Part model, mm, in its own coordinate system. A direction names the side the tool comes from. Give positions to 0.01 mm unless a question says otherwise; leave off trailing zeros. Order: outer loops, then holes, each group sorted by start corner. A loop starts at its lowest first (then second) coordinate and runs counter-clockwise, first axis right, second up. Notation, with made-up numbers: (7, -3) - (19, -3) arc R15 cw to (19, 8) - close; hole circle Ø2 at (71.5, 9.25). An arc over 180 degrees is marked (long way). Use a Markdown table: item, result. Add a question column.
Autodesk Inventor part; units mm, degrees
ref_plane "YZ Plane" through (0, 0, 0) normal (1, 0, 0) x (0, 1, 0)
ref_plane "XZ Plane" through (0, 0, 0) normal (0, 1, 0) x (-1, 0, 0)
ref_plane "XY Plane" through (0, 0, 0) normal (0, 0, 1) x (1, 0, 0)
sketch "Sketch1" plane through (0, 0, 0) normal (0, 0, 1) x (1, 0, 0)
  line L0 (0, 0) -> (19.4056, 0)
  line L1 (0, 0) -> (0, 19.05)
  line L2 (0, 19.05) -> (3.175, 19.05)
  line L3 (3.175, 0) -> (3.175, 3.175)
  line L4 (3.175, 3.175) -> (3.175, 19.05)
  line L5 (3.175, 3.175) -> (9.6266, 3.175)
  line L6 (9.6266, 3.175) -> (9.6266, 0)
  line L7 (19.2532, 0) -> (19.2532, 19.05)
  line L8 (19.2532, 19.05) -> (16.0782, 19.05)
  line L9 (16.0782, 3.175) -> (16.0782, 19.05)
  line L10 (16.0782, 3.175) -> (9.6266, 3.175)
  dimension "d0" = 19.4056
  dimension "d1" = 19.05
  dimension "d2" = 3.175
  dimension "d4" = 3.175
  dimension "d5" = 6.4516
extrude "Extrusion1" add sketch "Sketch1" along normal blind 12.7
sketch "Sketch2" plane through (3.175, 3.175, 0) normal (0, 1, 0) x (1, 0, 0)
  line L0 (12.9032, 0) -> (0, 0)
  line L1 (0, 0) -> (0, -12.7)
  line L2 (12.9032, -12.7) -> (0, -12.7)
  line L3 (12.9032, 0) -> (12.9032, -12.7)
  line L4 (0, 0) -> (6.4516, 0)
  line L5 (12.9032, 0) -> (0, 0)
  line L6 (6.4516, 0) -> (6.4516, -6.35)
  circle A0 centre (6.4516, -6.35) radius 2.3241
  point P0 (-3.175, 0)
  dimension "d8" = 6.4516
  dimension "d9" = 6.35
  dimension "d10" = 4.6482
extrude "Extrusion2" cut sketch "Sketch2" against normal blind 12.7 contours A0
chamfer "Chamfer1" distance 1.5875 angle 45 4 edges at (1.5875, 19.05, 0) (1.5875, 19.05, 12.7) (17.6657, 19.05, 12.7) (17.6657, 19.05, 0)
sketch "Sketch3" plane through (19.2532, 0, 12.7) normal (1, 0, 0) x (0, 0, -1)
  line L0 (11.1125, 19.05) -> (12.7, 17.4625)
  line L1 (11.1125, 19.05) -> (1.5875, 19.05)
  line L2 (0, 17.4625) -> (1.5875, 19.05)
  line L3 (0, 0) -> (0, 17.4625)
  line L4 (12.7, 0) -> (0, 0)
  line L5 (12.7, 0) -> (12.7, 17.4625)
  line L6 (12.7, 0) -> (0, 0)
  line L7 (12.7, 0) -> (6.35, 0)
  line L8 (6.35, 0) -> (6.35, 12.7)
  circle A0 centre (6.35, 12.7) radius 2.3241
  dimension "d16" = 6.35
  dimension "d17" = 12.7
  dimension "d18" = 4.6482
extrude "Extrusion3" cut sketch "Sketch3" against normal through all contours A0
fillet "Fillet1" radius 1.27 4 edges at (3.175, 3.175, 6.35) (16.0782, 3.175, 6.35) (19.2532, 0, 6.35) (0, 0, 6.35)
properties part number "U Bracket"
1. Tool access for faces 1 (the face through (19.253, 10, 6)), 2 (the face through (16.078, 10, 6)): list every direction of +Z, -Z, +X, -X, +Y, -Y with a clear straight run to the whole face (end or side of a thin tool).
2. Cut at C-C (y = 12.7). Write the cut outline in (x, z) (3 decimals), plus the area to 3 significant figures.
3. Drill centre lines: probe 1 along X at (y, z) = (9, 2.75) (3 decimals); probe 2 along Z at (x, y) = (17.3, 12.7); probe 3 along Y at (x, z) = (17.3, 6.35). Where is each one in solid material? Low to high. Write a range as [from, to].
4. Mould opens along Z. For faces 3 (the face through (17.688, 18.267, 0.805)), 4 (the face through (18, 19.05, 6)), 5 (the face through (1.61, 10.43, 6.85)), 6 (the face through (9.12, 1.61, 8.62)) say: released by +Z, released by -Z, zero draft, split by the parting line, or undercut.
5. Cut at A-A (z = 6.35). State how many separate pieces and enclosed holes the cut face has, plus the area to 3 significant figures.
6. Cut at B-B (y = 5.75). Write the cut outline in (x, z) (3 decimals).
7. Pin check, flat tip, straight feed: P1, Ø4, axis at y = 12.7, z = 6.35, coming from the -X side. Stop position of the tip, or through.
8. Cut at D-D (x = 8.5). Write the cut outline in (y, z) (3 decimals).
Responses:
| question | item | result |
|---|---|---|
| 1 | face 1 | +Z, -Z, +X, +Y, -Y |
| 1 | face 2 | +Z, -Z, +Y |
| 2 | outline | (0, 0) - (3.175, 0) - (3.175, 4.026) - (0, 4.026) - close; (0, 8.674) - (3.175, 8.674) - (3.175, 12.7) - (0, 12.7) - close; (16.078, 0) - (19.253, 0) - (19.253, 4.026) - (16.078, 4.026) - close; (16.078, 8.674) - (19.253, 8.674) - (19.253, 12.7) - (16.078, 12.7) - close |
| 2 | area | 51.1 mm² |
| 3 | probe 1 | x = [0, 3.175], [16.078, 19.253] |
| 3 | probe 2 | z = [0, 4.03], [8.67, 12.7] |
| 3 | probe 3 | y = [0, 10.38], [15.02, 19.05] |
| 4 | face 3 | released by -Z |
| 4 | face 4 | zero draft |
| 4 | face 5 | undercut |
| 4 | face 6 | undercut |
| 5 | separate pieces | 4 |
| 5 | enclosed holes | 0 |
| 5 | area | 118 mm² |
| 6 | outline | (0, 0) - (3.175, 0) - (3.175, 12.7) - (0, 12.7) - close; (16.078, 0) - (19.253, 0) - (19.253, 12.7) - (16.078, 12.7) - close |
| 7 | P1 | passes through |
| 8 | outline | (0, 0) - (3.175, 0) - (3.175, 4.317) - (0, 4.317) - close; (0, 8.383) - (3.175, 8.383) - (3.175, 12.7) - (0, 12.7) - close |
